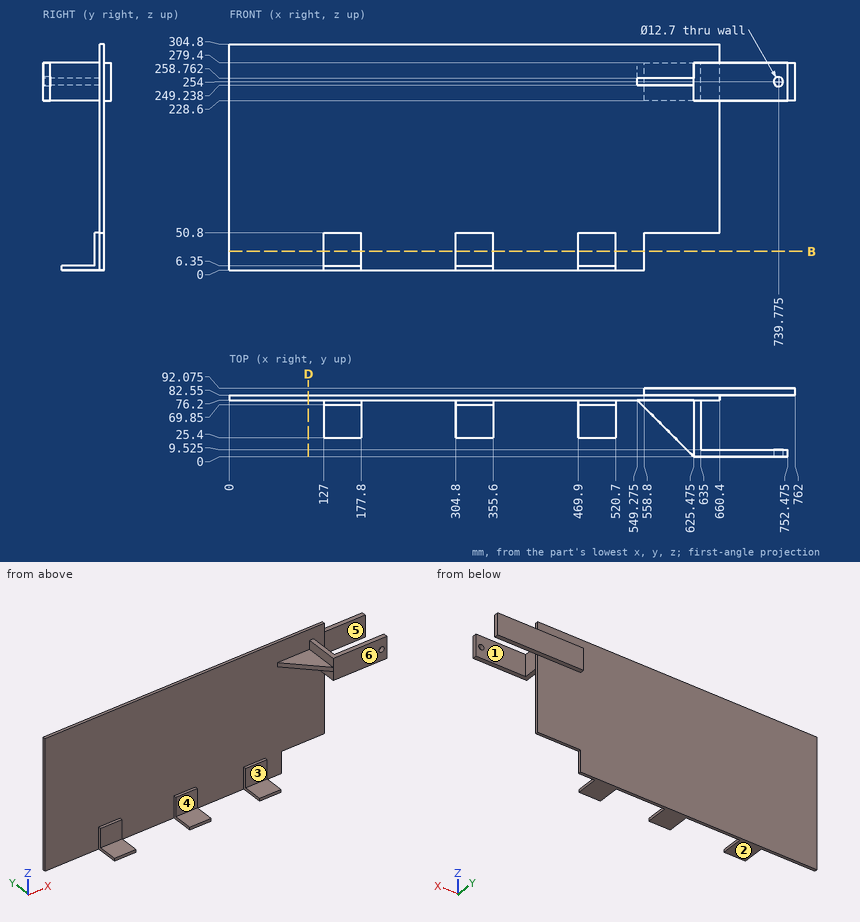
Can you work these out from the drawing? Everything is in mm from the part's minimum corner. A direction names the side the tool comes from. Coordinates: 2 decimals unless noted, no trailing zeros. Loops run counter-clockwise (first coordinate to the right, second up) from the corner with the lowest first, then second, coordinate; pieces in that order, holes last. Notation, with made-up numbers: M -36,-5.75 L -10,-5.75 A14 ccw -10,9.25 Z; hole C 36,-34 d7. An arc over 180 degrees is marked long. One line per item, written item: value.
1. Will these pins go through, and if not, where does the flat tip stop? pin 1 Ø22 at (x, z) = (153.5, 26) entering from -Y; pin 2 Ø7 at (x, y) = (500.5, 72.5) entering from +Z; pin 3 Ø22 at (x, y) = (322.5, 48.5) entering from +Z.
Geometry says:
pin 1: stops at y = 69.85
pin 2: stops at z = 50.8
pin 3: stops at z = 6.35
2. Please list where these lines run through material, in increasing order: probe 1 along Z at (x, y) = (327.5, 45); probe 2 along Y at (x, z) = (584.5, 203.5); probe 3 along X at (y, z) = (82, 186).
Geometry says:
probe 1: z = 0 to 6.35
probe 2: y = 76.2 to 82.55
probe 3: x = 0 to 660.4
3. Thinking about a two-plate mould opening in Y: for the marked faces 1, 2 and 3, which applies, +Y half, -Y half, draft (parallel to the pull), parting line (faces both ways), or undercut?
Geometry says:
face 1: undercut
face 2: draft
face 3: -Y half
4. Imagine slicing it at D-D (x = 106.5). List the corners of the cut face in (y, z) for me.
Geometry says:
outline: M 76.2,0 L 82.55,0 L 82.55,304.8 L 76.2,304.8 Z
5. Imagine slicing it at B-B (z = 25.5). List the corners of the cut face in (x, y) for me.
Geometry says:
outline: M 0,76.2 L 127,76.2 L 127,69.85 L 177.8,69.85 L 177.8,76.2 L 304.8,76.2 L 304.8,69.85 L 355.6,69.85 L 355.6,76.2 L 469.9,76.2 L 469.9,69.85 L 520.7,69.85 L 520.7,76.2 L 558.8,76.2 L 558.8,82.55 L 0,82.55 Z
6. On a 3-axis mill with a long thin cutter (end or side, diameter ignored), from which of +Z, -Z, +X, -X, +Y, -Y can I reach the whole of each face in a straight line? I mean the marked faces 4, 5 and 6. Say none if no direction works.
Geometry says:
face 4: +Z, +X, -X, -Y
face 5: +Z, -Z, +X
face 6: +Z, -Z, +X, -X, -Y
